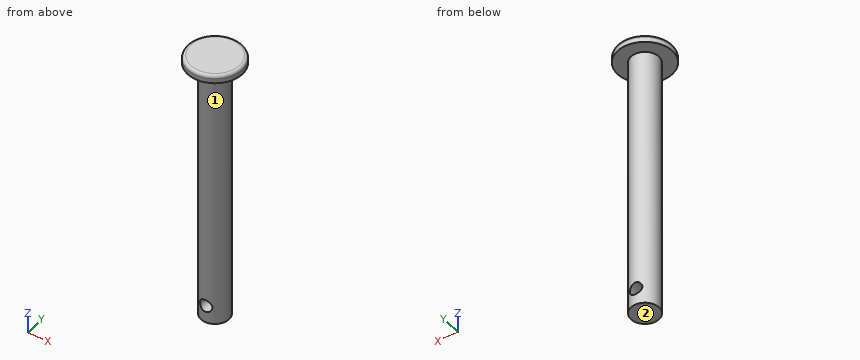
from build123d import *

# Parameters (mm, degrees)
IZIM1_R                     = 17.5
Y_KSEKLIK_EKSTR_ZYON1_DEPTH = 5
RADYUS1_R                   = 2
IZIM2_R                     = 9
Y_KSEKLIK_EKSTR_ZYON2_DEPTH = 170
IZIM3_R                     = 4
KES_EKSTR_ZYON1_DEPTH       = 85


with BuildPart() as part:
    # Çizim1 → Yükseklik-Ekstrüzyon1 (new body)
    with BuildSketch(Plane.XY):
        Circle(IZIM1_R)
    extrude(amount=Y_KSEKLIK_EKSTR_ZYON1_DEPTH)

    # Radyus1
    radyus1_edges = [part.edges().sort_by_distance(p)[0] for p in [
        (-17.5, 0, 5),
    ]]
    fillet(radyus1_edges, radius=RADYUS1_R)

    # Çizim2 → Yükseklik-Ekstrüzyon2 (add)
    with BuildSketch(Plane(origin=(0, 0, 0), x_dir=(-1, 0, 0), z_dir=(0, 0, -1))):
        Circle(IZIM2_R)
    extrude(amount=Y_KSEKLIK_EKSTR_ZYON2_DEPTH)

    # Çizim3 → Kes-Ekstrüzyon1 (cut, symmetric)
    with BuildSketch(Plane(origin=(0, 0, 0), x_dir=(1, 0, 0), z_dir=(0, 1, 0))):
        with Locations((0, 159)):
            Circle(IZIM3_R)
    extrude(amount=KES_EKSTR_ZYON1_DEPTH, both=True, mode=Mode.SUBTRACT)


solid = part.part
Input: part model. Units: mm. Frame: model coordinates. Face numbers are marked on the shaded views. A direction names the side the tool comes from. Coordinates: 2 decimals unless noted, no trailing zeros. Loops run counter-clockwise (first coordinate to the right, second up) from the corner with the lowest first, then second, coordinate; pieces in that order, holes last. Notation, with made-up numbers: (-7.75, 56) - (7.25, 56) arc R18 ccw to (7.25, 77) - close; hole circle Ø4 at (-19, 62.5). An arc over 180 degrees is marked (long way). Answer in a Markdown table with one row per item. Add a question column.
Item 1: Section query A-A on x = 0. Return the cut outline in (y, z).
Item 2: Section query B-B on y = 0. Return the cut outline in (x, z).
Item 3: Contact query for flat-ended pins moving along their axis: P1, Ø12, axis at x = -10.5, z = -77.5, coming from the -Y side; P2, Ø10, axis at x = 10, z = -35, coming from the -Y side; P3, Ø6, axis at x = -9, y = -4, coming from the -Z side; P4, Ø12, axis at x = -2, z = -76, coming from the +Y side. Output: stop coordinate, or through.
Item 4: Section query C-C on z = -159. Return the cut outline in (x, y), then the cut area to 3 significant figures.
Item 5: Access query for the marked faces 1 and 2. Directions: +Z, -Z, +X, -X, +Y, -Y. A direction counts if a zero-diameter tool reaches every point of the face in a straight line with its end or side. Return the directions, or none.
Item 6: Line query: line 1 along Z through (x, y) = (0, 2.5); line 2 along Z through (x, y) = (-5.5, 14); line 3 along X through (y, z) = (-3, -159). Output: solid intervals per line, ascending. Write a range as [from, to].
Recorded:
| question | item | result |
|---|---|---|
| 1 | outline | (-17.5, 0) - (-9, 0) - (-9, -155) - (9, -155) - (9, 0) - (17.5, 0) - (17.5, 3) arc R2 ccw to (15.5, 5) - (-15.5, 5) arc R2 ccw to (-17.5, 3) - close; (-9, -170) - (9, -170) - (9, -163) - (-9, -163) - close |
| 2 | outline | (-17.5, 0) - (-9, 0) - (-9, -170) - (9, -170) - (9, 0) - (17.5, 0) - (17.5, 3) arc R2 ccw to (15.5, 5) - (-15.5, 5) arc R2 ccw to (-17.5, 3) - close; hole circle Ø8 at (0, -159) |
| 3 | P1 | y = -7.79 |
| 3 | P2 | y = -7.48 |
| 3 | P3 | z = -170 |
| 3 | P4 | y = 9 |
| 4 | outline | (-4, -8.06) - (-4, 8.06) arc R9 ccw to start; (4, -8.06) arc R9 ccw to (4, 8.06) - close |
| 4 | area | 115 mm^2 |
| 5 | face 1 | -Z |
| 5 | face 2 | -Z, +X, -X, +Y, -Y |
| 6 | line 1 | [-170, -163], [-155, 5] |
| 6 | line 2 | [0, 5] |
| 6 | line 3 | [-8.49, -4], [4, 8.49] |
